```python
from build123d import *

# Parameters (mm, degrees)
SKETCH_1_W          = 80
SKETCH_1_H          = 45
EXTRUDE_1_DEPTH     = 3
SKETCH_2_R          = 1.65
CUT_EXTRUDE_1_DEPTH = 3
SKETCH_3_R          = 13
CUT_EXTRUDE_2_DEPTH = 10
SKETCH_5_R          = 1.7
CUT_EXTRUDE_4_DEPTH = 10


with BuildPart() as part:
    # 草图1 → 凸台-拉伸1 (new body)
    with BuildSketch(Plane(origin=(0, 0, 0), x_dir=(1, 0, 0), z_dir=(0, 1, 0))):
        Rectangle(SKETCH_1_W, SKETCH_1_H)
    extrude(amount=EXTRUDE_1_DEPTH)

    # 草图2 → 切除-拉伸1 (cut)
    with BuildSketch(Plane(origin=(0, 3, 0), x_dir=(1, 0, 0), z_dir=(0, 1, 0))):
        with Locations(Location((-15.5, 15.5, 0), (0, 0, 270))):
            Circle(SKETCH_2_R)
        with Locations(Location((15.5, 15.5, 0), (0, 0, 270))):
            Circle(SKETCH_2_R)
        with Locations(Location((-15.5, -15.5, 0), (0, 0, 270))):
            Circle(SKETCH_2_R)
        with Locations(Location((15.5, -15.5, 0), (0, 0, 270))):
            Circle(SKETCH_2_R)
    extrude(amount=-CUT_EXTRUDE_1_DEPTH, mode=Mode.SUBTRACT)

    # 草图3 → 切除-拉伸2 (cut)
    with BuildSketch(Plane(origin=(0, 3, 0), x_dir=(1, 0, 0), z_dir=(0, 1, 0))):
        with Locations(Location((0, 0, 0), (0, 0, 270))):
            Circle(SKETCH_3_R)
    extrude(amount=-CUT_EXTRUDE_2_DEPTH, mode=Mode.SUBTRACT)

    # 草图5 → 切除-拉伸4 (cut)
    with BuildSketch(Plane(origin=(0, 3, 0), x_dir=(1, 0, 0), z_dir=(0, 1, 0))):
        with Locations(Location((-30, 15, 0), (0, 0, 270))):
            Circle(SKETCH_5_R)
        with Locations(Location((30, 15, 0), (0, 0, 90))):
            Circle(SKETCH_5_R)
        with Locations(Location((-30, -15, 0), (0, 0, 90))):
            Circle(SKETCH_5_R)
        with Locations(Location((30, -15, 0), (0, 0, 270))):
            Circle(SKETCH_5_R)
    extrude(amount=-CUT_EXTRUDE_4_DEPTH, mode=Mode.SUBTRACT)


solid = part.part
```
Geometry check sheet. Reference: the model listing, model coordinates, mm. Round coordinates to 2 decimals unless told otherwise and drop trailing zeros. Order: outer loops, then holes, each group sorted by start corner. A loop starts at its lowest first (then second) coordinate and runs counter-clockwise, first axis right, second up. Notation, with made-up numbers: M 41,47 L 72,47 A26 cw 72,71 Z; hole C 87.5,6.5 d1. An arc over 180 degrees is marked long. Write item = value, one per line.
Q1. Release check for a two-part mould opening along Z. For faces 1 (the flat face through (40, 1, 0)), 2 (the cylindrical face through (28.5, 1.5, 15.8)), 3 (the flat face through (-1, 1, 22.5)) record: released by +Z, released by -Z, zero draft, split by the parting line, or undercut.
Answer block:
face_1 = zero draft
face_2 = undercut
face_3 = released by +Z
Q2. Section check D-D (x = -5). Enter the section's corners in (y, z), plus the area to 3 significant figures.
Answer block:
outline = M 0,-22.5 L 3,-22.5 L 3,-12 L 0,-12 Z; M 0,12 L 3,12 L 3,22.5 L 0,22.5 Z
area = 63.0 mm^2
Q3. Section check A-A (y = 1.25). Give the number of separate pieces and of enclosed holes in the cut face, plus the area to 3 significant figures.
Answer block:
separate_pieces = 1
enclosed_holes = 9
area = 3,000 mm^2
Q4. Section check C-C (z = 0). Enter the section's corners in (x, y).
Answer block:
outline = M -40,0 L -13,0 L -13,3 L -40,3 Z; M 13,0 L 40,0 L 40,3 L 13,3 Z
Q5. Scan lines: line 1 (X direction, y = 0.85, z = -14); line 2 (X direction, y = 2.3, z = 15.5); line 3 (X direction, y = 0.35, z = -0.5). Record each from-to range of solid material in increasing order.
Answer block:
line_1 = -40 to -31.37, -28.63 to -16.19, -14.81 to 14.81, 16.19 to 28.63, 31.37 to 40
line_2 = -40 to -31.62, -28.38 to -17.15, -13.85 to 13.85, 17.15 to 28.38, 31.62 to 40
line_3 = -40 to -12.99, 12.99 to 40
Q6. Section check B-B (x = -30). Enter the section's corners in (y, z).
Answer block:
outline = M 0,-22.5 L 3,-22.5 L 3,-16.7 L 0,-16.7 Z; M 0,-13.3 L 3,-13.3 L 3,13.3 L 0,13.3 Z; M 0,16.7 L 3,16.7 L 3,22.5 L 0,22.5 Z
